Geometry: final body of the model. Coordinates: model frame, mm. A direction names the side the tool comes from. Give positions to 0.01 mm unless a question says otherwise; leave off trailing zeros. Write each loop counter-clockwise with the first axis right and the second up, starting at its lowest first coordinate (ties: lowest second). Pieces come first, ordered by that corner, then holes.
Q1. Section D-D (y = -5.5). State how many separate pieces and enclosed holes the cut face has, plus the area to 4 significant figures.
Q2. Mould query, pull axis Y, two halves, no side actions, for faces 4 (the flat face through (1, -0.5, -1)), 5 (the cylindrical face through (9.78, -5.02, -16.95)), 6 (the flat face through (4, 2, -27.475)). Classes: +Y half, -Y half, draft (parallel to the pull), parting line (faces both ways), or undercut.
Q3. Section C-C (z = 17). Return the cut outline in (x, y).
Q4. Line query: line 1 (X direction, y = -5.5, z = -1); line 2 (X direction, y = -1, z = 0.5); line 3 (Z direction, x = 1.75, y = 4.25) (3 decimals). Output: solid intervals per line, ascending.
Q5. Pin query (flat end, axial travel): pin 1 Ø1 at (x, z) = (5.5, 0.5) entering from +Y; pin 2 Ø5 at (x, z) = (5.5, -6.5) entering from -Y; pin 3 Ø2 at (x, z) = (4.5, -10) entering from -Y. Return the tip coordinate at first contact, or that it passes through.
Q6. Section A-A (z = -16). Return the cut outline in (x, y).
Q7. Reachability of faces 1 (the cylindrical face through (9.78, -5.02, 13.05)), 2 (the flat face through (6, -2, -1)), 3 (the flat face through (4, 2, 25.525)) from +Z, -Z, +X, -X, +Y, -Y: full face, straight path, thin tool, end or side. Return the list, or none.
Q8. Section B-B (y = 1.75). Return the cut outline in (x, z) (3 decimals), plus the area to 3 significant figures.
Autodesk Inventor part; units mm, degrees
ref_plane "YZ Plane" through (0, 0, 0) normal (1, 0, 0) x (0, 1, 0)
ref_plane "XZ Plane" through (0, 0, 0) normal (0, 1, 0) x (-1, 0, 0)
ref_plane "XY Plane" through (0, 0, 0) normal (0, 0, 1) x (1, 0, 0)
sketch "Sketch1" plane through (0, 0, 0) normal (0, 1, 0) x (-1, 0, 0)
  line L0 (2.7098, 27.525) -> (-10.7902, 27.525)
  line L1 (-10.7902, 27.525) -> (-10.7902, -29.475)
  line L2 (-10.7902, -29.475) -> (2.7098, -29.475)
  line L3 (2.7098, -29.475) -> (2.7098, 27.525)
  line L4 (-4.0402, 27.525) -> (-4.0402, -29.475)
  line L5 (0.7098, 27.525) -> (0.7098, -29.475)
  line L6 (-8.7902, 27.525) -> (-8.7902, -29.475)
  line L7 (-8.7902, 27.525) -> (-10.7902, 27.525)
  line L8 (-10.7902, 27.525) -> (-10.7902, -29.475)
  line L9 (-10.7902, -29.475) -> (-8.7902, -29.475)
  line L10 (-8.7902, -29.475) -> (-8.7902, 27.525)
  line L11 (2.7098, -29.475) -> (0.7098, -29.475)
  line L12 (0.7098, -29.475) -> (0.7098, 27.525)
  line L13 (0.7098, 27.525) -> (2.7098, 27.525)
  line L14 (2.7098, 27.525) -> (2.7098, -29.475)
  dimension "d31" = 57
  dimension "d33" = 2
  dimension "d34" = 9.5
extrude "Extrusion6" add sketch "Sketch1" along normal blind 5 contours L3 L2 L5 L0 | L6 L2 L1 L0
extrude "Extrusion7" add sketch "Sketch1" against normal blind 2
sketch "Sketch4" plane through (-2.7098, 5, -29.475) normal (-1, 0, 0) x (0, 0, 1)
  line L0 (57, -7) -> (57, 0) construction
  line L1 (0, 0) -> (57, 0) construction
  line L2 (0, -7) -> (0, 0) construction
  line L3 (57, -7) -> (0, -7) construction
  line L4 (55, 0) -> (2, 0)
  line L5 (2, 0) -> (2, -5.5)
  line L6 (2, -5.5) -> (55, -5.5)
  line L7 (55, -5.5) -> (55, 0)
  point P0 (29.475, -5)
  dimension "d39" = 2
  dimension "d40" = 2
  dimension "d41" = 1.5
extrude "Extrusion8" cut sketch "Sketch4" against normal up to surface (13.5 mm away)
sketch "Sketch5" plane through (8.7902, 0, 27.525) normal (-1, 0, 0) x (0, 0, 1)
  line L0 (-2, 5) -> (-2, 0)
  line L1 (-2, 0) -> (0, 0)
  line L2 (0, 0) -> (0, 5)
  line L3 (-2, 5) -> (0, 5)
  line L4 (-55, 0) -> (-55, 5)
  line L5 (-57, 5) -> (-55, 5)
  line L6 (-57, 0) -> (-57, 5)
  line L7 (-57, 0) -> (-55, 0)
  point P0 (-27.525, 0)
extrude "Extrusion9" add sketch "Sketch5" along normal through all both and the other way through all
sketch "Sketch6" plane through (0, -2, 0) normal (0, -1, 0) x (1, 0, 0)
  line L0 (10.7902, 27.525) -> (-2.7098, 27.525) construction
  line L1 (-2.7098, 27.525) -> (-2.7098, -29.475) construction
  line L2 (-2.7098, -29.475) -> (10.7902, -29.475) construction
  line L3 (10.7902, -29.475) -> (10.7902, 27.525) construction
  line L4 (4.0402, 32.9205) -> (4.0402, -29.475)
  line L5 (5.6402, 24.1195) -> (2.4402, 24.1195)
  line L6 (2.4402, 24.1195) -> (2.4402, -25.8805)
  line L7 (2.4402, -25.8805) -> (5.6402, -25.8805)
  line L8 (5.6402, -25.8805) -> (5.6402, 24.1195)
  point P0 (0, 0)
  dimension "d46" = 50
  dimension "d47" = 3.2
extrude "Extrusion10" cut sketch "Sketch6" against normal through all
sketch "Sketch7" plane through (0, -2, 0) normal (0, -1, 0) x (1, 0, 0)
  line L0 (2.4402, -25.8805) -> (2.4402, 24.1195) construction
  line L1 (2.4402, 24.1195) -> (5.6402, 24.1195) construction
  line L2 (5.6402, 24.1195) -> (5.6402, -25.8805) construction
  line L3 (5.6402, -25.8805) -> (2.4402, -25.8805) construction
  line L4 (10.7902, 27.525) -> (-2.7098, 27.525) construction
  line L5 (-2.7098, 27.525) -> (-2.7098, -29.475) construction
  line L6 (-2.7098, -29.475) -> (10.7902, -29.475) construction
  line L7 (10.7902, -29.475) -> (10.7902, 27.525) construction
  line L8 (-2.7098, 27.525) -> (-0.7098, 27.525)
  line L9 (-0.7098, 27.525) -> (-0.7098, -29.475)
  line L10 (-0.7098, -29.475) -> (-2.7098, -29.475)
  line L11 (-2.7098, -29.475) -> (-2.7098, 27.525)
  line L12 (10.7902, 27.525) -> (8.7902, 27.525)
  line L13 (8.7902, 27.525) -> (8.7902, -29.475)
  line L14 (8.7902, -29.475) -> (10.7902, -29.475)
  line L15 (10.7902, -29.475) -> (10.7902, 27.525)
  line L16 (-2.7098, -29.475) -> (10.7902, -29.475)
  point P0 (0, 0)
  dimension "d50" = 2
  dimension "d51" = 2
extrude "Extrusion11" add sketch "Sketch7" along normal blind 7
sketch "Sketch8" plane through (-2.7098, -0.5, 25.525) normal (-1, 0, 0) x (0, 0, 1)
  line L0 (2, -8.5) -> (2, 5.5) construction
  line L1 (0, 5.5) -> (2, 5.5) construction
  line L2 (0, 5.5) -> (0, 0) construction
  line L3 (0, 0) -> (-53, 0) construction
  line L4 (-53, 0) -> (-53, 5.5) construction
  line L5 (-55, 5.5) -> (-53, 5.5) construction
  line L6 (-55, -8.5) -> (-55, 5.5) construction
  line L7 (2, -8.5) -> (-55, -8.5) construction
  line L8 (-55, -8.5) -> (-55, 5.5) construction
  line L9 (2, -8.5) -> (-55, -8.5) construction
  line L10 (-55, -8.5) -> (-55, 0) construction
  line L11 (-55, 0) -> (2, 0) construction
  line L12 (2, 0) -> (2, -8.5) construction
  circle A0 centre (-4, -5) radius 1.6
  point P0 (-25.525, 0.5)
  dimension "d54" = 3.2
  dimension "d55" = 5
  dimension "d56" = 6
extrude "Extrusion12" cut sketch "Sketch8" against normal through all
pattern_linear "Rectangular Pattern3" count 10 spacing 5 along (0, 0, -1) of "Extrusion12"
properties part number "slider-rail-adapter"
Computed:
1. separate pieces: 22
1. enclosed holes: 0
1. area: 100.0 mm2
2. face 4: +Y half
2. face 5: undercut
2. face 6: draft
3. outline: (-2.71, -9) - (-0.71, -9) - (-0.71, -7.03) - (-2.71, -7.03) - close; (-2.71, -3.97) - (-0.71, -3.97) - (-0.71, -2) - (2.44, -2) - (2.44, -0.5) - (-2.71, -0.5) - close; (5.64, -2) - (8.79, -2) - (8.79, -3.97) - (10.79, -3.97) - (10.79, -0.5) - (5.64, -0.5) - close; (8.79, -9) - (10.79, -9) - (10.79, -7.03) - (8.79, -7.03) - close
4. line 1: x = -2.71 to -0.71, 8.79 to 10.79
4. line 2: x = -2.71 to 2.44, 5.64 to 10.79
4. line 3: z = -29.475 to -27.475, 25.525 to 27.525
5. pin 1: stops at y = -0.5
5. pin 2: stops at y = -2
5. pin 3: passes through
6. outline: (-2.71, -9) - (-0.71, -9) - (-0.71, -2) - (2.44, -2) - (2.44, -0.5) - (-2.71, -0.5) - close; (5.64, -2) - (8.79, -2) - (8.79, -9) - (10.79, -9) - (10.79, -0.5) - (5.64, -0.5) - close
7. face 1: +X, -X
7. face 2: +Z, -Z, -Y
7. face 3: +X, -X, +Y
8. outline: (-2.71, -29.475) - (10.79, -29.475) - (10.79, -27.475) - (-2.71, -27.475) - close; (-2.71, 25.525) - (10.79, 25.525) - (10.79, 27.525) - (-2.71, 27.525) - close
8. area: 54.0 mm2
